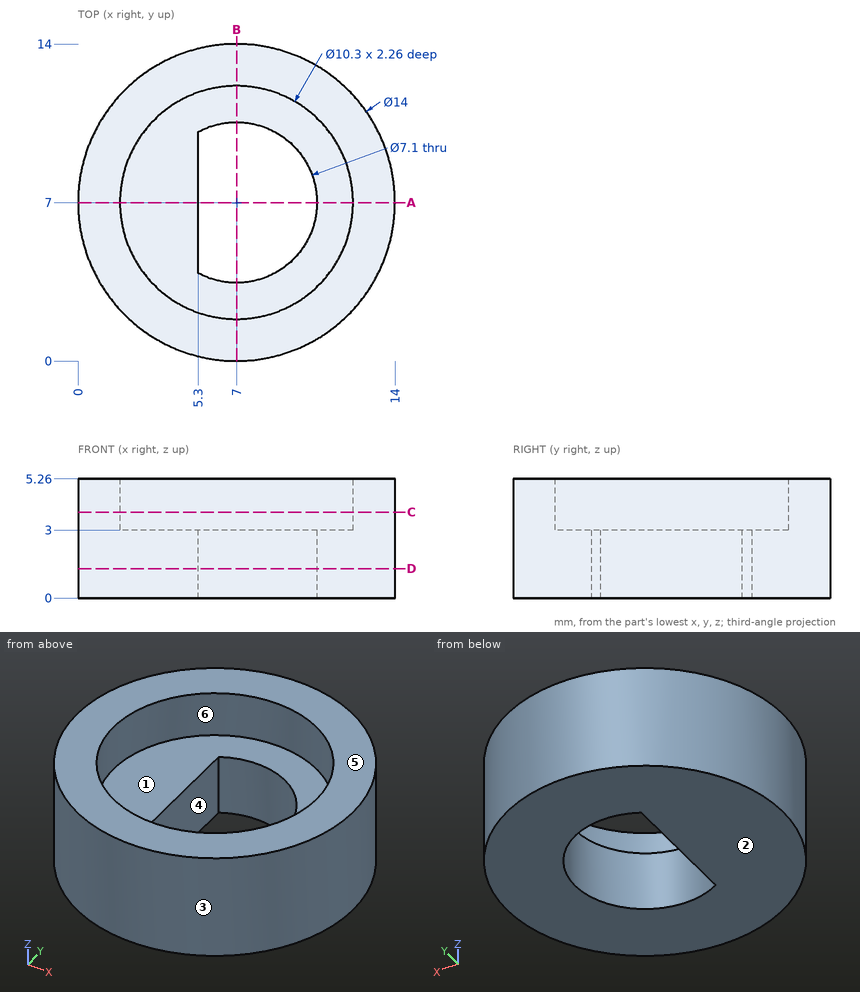
Job drawing, mm, ordinate dimensions from the low corner. One solid piece. A direction names the side the tool comes from. Round coordinates to 2 decimals unless told otherwise and drop trailing zeros. Write each loop counter-clockwise with the first axis right and the second up, starting at its lowest first coordinate (ties: lowest second). Pieces come first, ordered by that corner, then holes. Notation, with made-up numbers: M -33,-14.75 L -21,-14.75 A10 cw -21,-10.75 Z; hole C 41.25,-10 d7. An arc over 180 degrees is marked long. Return JSON: item names as keys, results as strings. Group by question number.
(1) Saw through at B-B on x = 7. Write the cut outline in (y, z).
(2) Saw through at A-A on y = 7. Write the cut outline in (x, z), then the cut area to 3 significant figures.
(3) Two-plate mould, pull along Y, no slides. Class the marked faces 1, 2 and 3: +Y half, -Y half, draft (parallel to the pull), parting line (faces both ways), or undercut.
(4) Saw through at D-D on z = 1.3. Write the cut outline in (x, y), then the cut area to 3 significant figures.
(5) Drill centre lines: probe 1 along Y at (x, z) = (7, 0.65); probe 2 along Y at (x, z) = (7, 4.7); probe 3 along X at (y, z) = (9.25, 3.55). Where is each one in solid material? Low to high.
(6) Pin check, flat tips, straight feed: pin 1 Ø1.5 at (y, z) = (6, 1) entering from +X; pin 2 Ø1 at (x, z) = (5.5, 2.5) entering from +Y; pin 3 Ø8 at (x, y) = (6.5, 7) entering from +Z. Stop position of each tip, or through.
(7) Saw through at C-C on z = 3.8. Write the cut outline in (x, y), then the cut area to 3 significant figures.
(8) Which spindle directions (+Z, -Z, +X, -X, +Y, -Y) get a long thin tool onto all of the face, cutting with end or side? Do the marked faces 4, 5 and 6. Say none if no direction does.
Returned:
{
 "1": {"outline": "M 0,0 L 3.45,0 L 3.45,3 L 1.85,3 L 1.85,5.26 L 0,5.26 Z; M 10.55,0 L 14,0 L 14,5.26 L 12.15,5.26 L 12.15,3 L 10.55,3 Z"},
 "2": {"outline": "M 0,0 L 5.3,0 L 5.3,3 L 1.85,3 L 1.85,5.26 L 0,5.26 Z; M 10.55,0 L 14,0 L 14,5.26 L 12.15,5.26 L 12.15,3 L 10.55,3 Z", "area": "34.6 mm²"},
 "3": {"face 1": "undercut", "face 2": "draft", "face 3": "parting line"},
 "4": {"outline": "C 7,7 d14; hole M 5.3,3.88 A3.55 ccw long 5.3,10.12 Z", "area": "123 mm²"},
 "5": {"probe 1": "0 to 3.45, 10.55 to 14", "probe 2": "0 to 1.85, 12.15 to 14", "probe 3": "0.37 to 2.37, 11.63 to 13.63"},
 "6": {"pin 1": "x = 14", "pin 2": "y = 13.93", "pin 3": "z = 3"},
 "7": {"outline": "C 7,7 d14; hole C 7,7 d10.3", "area": "70.6 mm²"},
 "8": {"face 4": "+Z, -Z", "face 5": "+Z, +X, -X, +Y, -Y", "face 6": "+Z"}
}
